Check sheet for the drawn part. Datum: minimum x, y, z corner. Units: mm. Give positions to 0.01 mm unless a question says otherwise; leave off trailing zeros. Order: outer loops, then holes, each group sorted by start corner. A loop starts at its lowest first (then second) coordinate and runs counter-clockwise, first axis right, second up. Notation, with made-up numbers: (61.5, 25.25) -> (106.5, 25.25) arc R25 cw to (106.5, 50.25) -> close; hole circle Ø7 at (35, 61). An arc over 180 degrees is marked (long way). Return JSON: item names as keys, results as strings. Group by question number.
(1) Cross-section at C-C on z = 1.25. Enter the section's corners in (x, y), then the cut area to 3 significant figures.
(2) Cross-section at A-A on x = 50. Enter the section's corners in (y, z).
(3) Thickness scan on line 1 along Y through (x, z) = (50, 6.75); line 2 along Y through (x, z) = (63, 4); line 3 along X through (y, z) = (46.5, 3). Record the ranges inside material, lowest first.
(4) Release check for a two-part mould opening along X. For the marked faces 1 and 2 record: pulls with the +X half, pulls with the -X half, needs draft (parallel to the pull), parting line crosses it, or undercut.
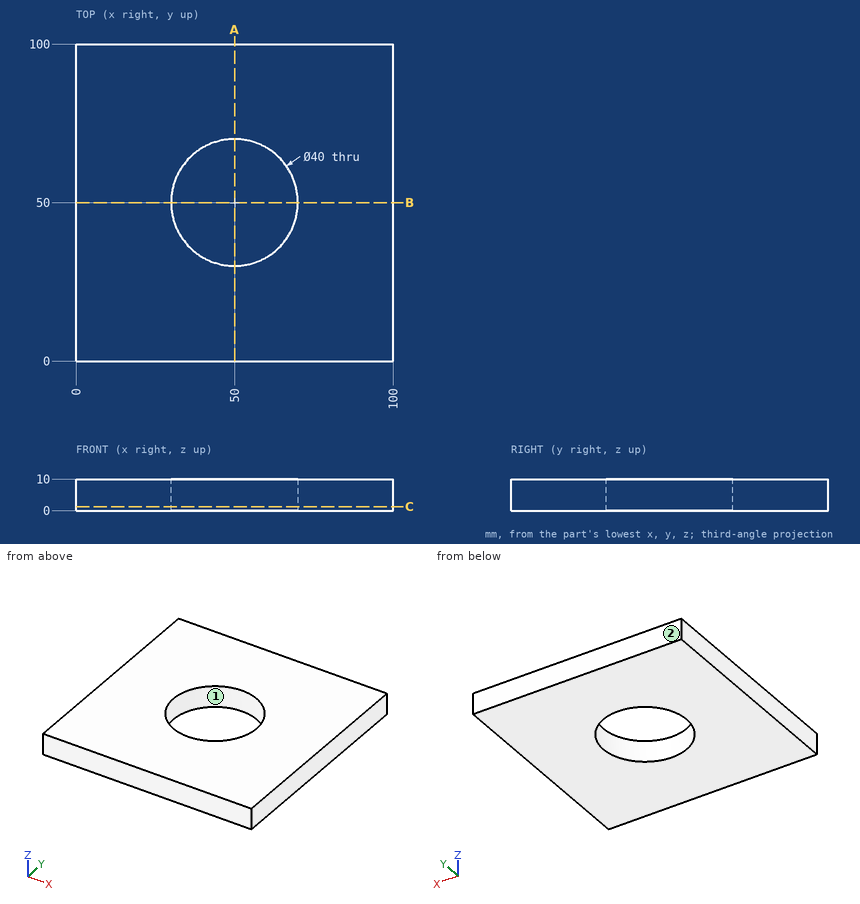
Verdict:
{
 "1": {"outline": "(0, 0) -> (100, 0) -> (100, 100) -> (0, 100) -> close; hole circle Ø40 at (50, 50)", "area": "8,740 mm²"},
 "2": {"outline": "(0, 0) -> (30, 0) -> (30, 10) -> (0, 10) -> close; (70, 0) -> (100, 0) -> (100, 10) -> (70, 10) -> close"},
 "3": {"line 1": "0 to 30, 70 to 100", "line 2": "0 to 34.8, 65.2 to 100", "line 3": "0 to 30.31, 69.69 to 100"},
 "4": {"face 1": "undercut", "face 2": "needs draft"}
}
